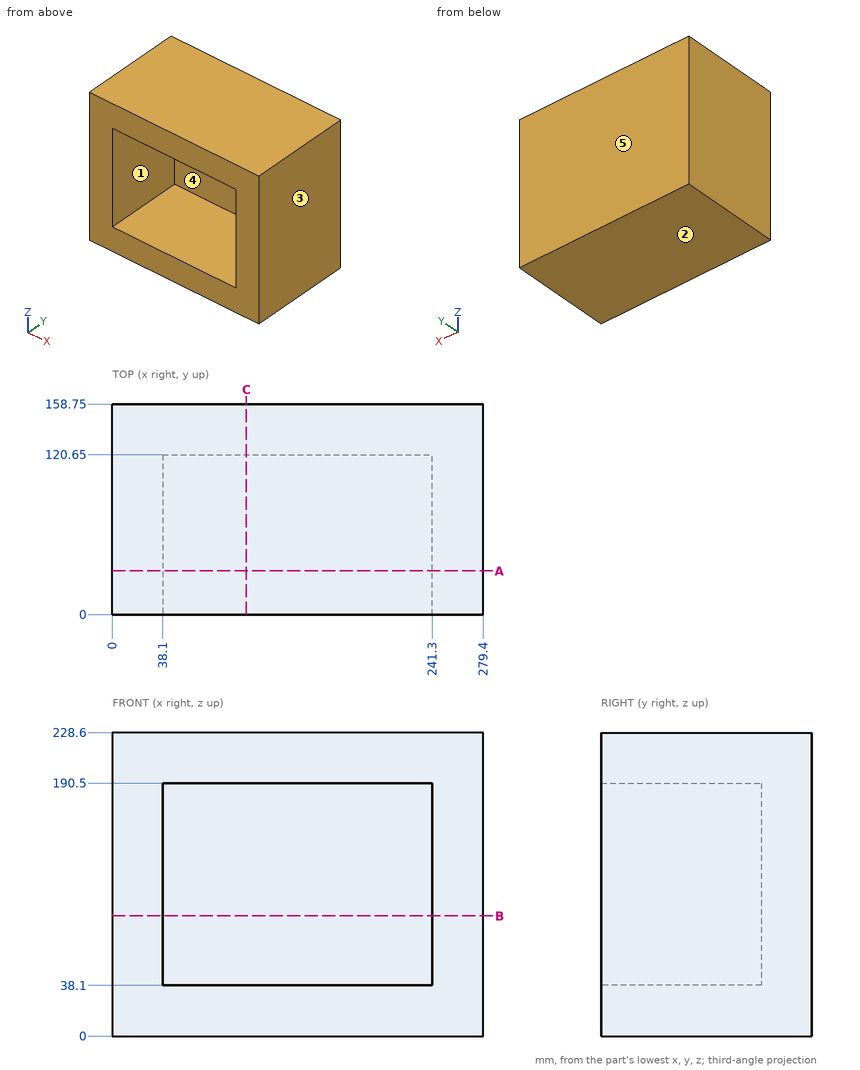
Geometry: see drawing. Coordinates: mm, zero at the bounding-box minimum. A direction names the side the tool comes from. Give positions to 0.01 mm unless a question says otherwise; leave off trailing zeros. Loops run counter-clockwise (first coordinate to the right, second up) from the corner with the lowest first, then second, coordinate; pieces in that order, holes last. Notation, with made-up numbers: (-18, -12.5) -> (7, -12.5) arc R14 cw to (7, -0.5) -> close; hole circle Ø5 at (-5.5, 56). An arc over 180 degrees is marked (long way). Use one line per item in the form item = value.
Item 1: Section query A-A on y = 33. Output: boundary loops of the cut face in (x, z), and give its area (3 significant figures).
A:
outline = (0, 0) -> (279.4, 0) -> (279.4, 228.6) -> (0, 228.6) -> close; hole (38.1, 38.1) -> (241.3, 38.1) -> (241.3, 190.5) -> (38.1, 190.5) -> close
area = 32,900 mm^2
Item 2: Section query C-C on x = 101. Output: boundary loops of the cut face in (y, z).
A:
outline = (0, 0) -> (158.75, 0) -> (158.75, 228.6) -> (0, 228.6) -> (0, 190.5) -> (120.65, 190.5) -> (120.65, 38.1) -> (0, 38.1) -> close
Item 3: Access query for the marked faces 1 and 2. Directions: +Z, -Z, +X, -X, +Y, -Y. A direction counts if a zero-diameter tool reaches every point of the face in a straight line with its end or side. Return the directions, or none.
A:
face_1 = -Y
face_2 = -Z, +X, -X, +Y, -Y
Item 4: Section query B-B on z = 90.5. Output: boundary loops of the cut face in (x, y).
A:
outline = (0, 0) -> (38.1, 0) -> (38.1, 120.65) -> (241.3, 120.65) -> (241.3, 0) -> (279.4, 0) -> (279.4, 158.75) -> (0, 158.75) -> close
Item 5: Draft query along X for the marked faces 3, 4 and 5. Return one class per face: pulls with the +X half, pulls with the -X half, needs draft (parallel to the pull), parting line crosses it, or undercut.
A:
face_3 = pulls with the +X half
face_4 = undercut
face_5 = needs draft
Item 6: Line query: probe 1 along X at (y, z) = (38.5, 172.5); probe 2 along Z at (x, y) = (167.5, 60.5); probe 3 along Y at (x, z) = (134, 119). Output: solid intervals per line, ascending.
A:
probe_1 = 0 to 38.1, 241.3 to 279.4
probe_2 = 0 to 38.1, 190.5 to 228.6
probe_3 = 120.65 to 158.75
